```python
from build123d import *

# Parameters (mm, degrees)
F0_R     = 9
F1_DEPTH = 27.2
F2_R     = 5.5
F3_DEPTH = 23.7
F4_SIZE  = 1.5


with BuildPart() as f1:
    # F0 (on Top) → F1 (new body)
    with BuildSketch(Plane.XY):
        Circle(F0_R)
    extrude(amount=-F1_DEPTH)

    # F2 (on face) → F3 (cut)
    with BuildSketch(Plane.XY):
        Circle(F2_R)
    extrude(amount=-F3_DEPTH, mode=Mode.SUBTRACT)

    # F4
    f4_edges = [f1.edges().sort_by_distance(p)[0] for p in [
        (-9, 0, 0),
    ]]
    chamfer(f4_edges, length=F4_SIZE)


solid = f1.part
```
The listing builds one solid part. Answer for the finished solid, in the listing's coordinates (mm). A direction names the side the tool comes from. Give positions to 0.01 mm unless a question says otherwise; leave off trailing zeros. Write each loop counter-clockwise with the first axis right and the second up, starting at its lowest first coordinate (ties: lowest second). Pieces come first, ordered by that corner, then holes. Notation, with made-up numbers: (3, 39.5) - (36, 39.5) arc R24 cw to (36, 51.5) - close; hole circle Ø9 at (33, 32.5). An arc over 180 degrees is marked (long way). Use one line per item in the form item = value. Start each with the question number.
1) Find section B-B on x = 0. Determine the outline of the cut face in (y, z).
2) A tool of negligible diameter and unlimited length cuts with its end or side. For faces 1 (the face through (-1.19, -5.37, -11.68)), 2 (the face through (-4, 4, 0)), from which of +Z, -Z, +X, -X, +Y, -Y can it reach the whole face along a straight path? Write none if from no direction.
3) The mould has two halves that part along Y. Classify faces 3 (the face through (-1.172, 8.923, -14.17)), 4 (the face through (0, 0, -23.7)), 5 (the face through (0, 0, -27.2)): pulls with the +Y half, pulls with the -Y half, needs draft (parallel to the pull), parting line crosses it, or undercut.
4) Consider line 1 along Y through (x, z) = (0, -13.5); line 2 along X through (y, z) = (4.5, -7.75); line 3 along Z through (x, y) = (5, -0.25). Determine where each line is inside the solid, lowest interval first. Write a range as from..to.
5) Find section A-A on z = -3. Determine the outline of the cut face in (x, y).
6) Flat-ended cylindrical pins translate along their axes: pin 1 Ø1.5 at (x, z) = (-3.5, -7) entering from -Y; pin 2 Ø6 at (y, z) = (7, -14) entering from +X; pin 3 Ø3 at (y, z) = (7, -22) entering from +X. Find the tip coordinate at first contact, or state that the pin passes through.
Geometry results:
q1.outline = (-9, -27.2) - (9, -27.2) - (9, -1.5) - (7.5, 0) - (5.5, 0) - (5.5, -23.7) - (-5.5, -23.7) - (-5.5, 0) - (-7.5, 0) - (-9, -1.5) - close
q2.face_1 = +Z
q2.face_2 = +Z, +X, -X, +Y, -Y
q3.face_3 = parting line crosses it
q3.face_4 = undercut
q3.face_5 = needs draft
q4.line_1 = -9..-5.5, 5.5..9
q4.line_2 = -7.79..-3.16, 3.16..7.79
q4.line_3 = -27.2..-23.7
q5.outline = circle Ø18 at (0, 0); hole circle Ø11 at (0, 0)
q6.pin_1 = -8.57
q6.pin_2 = 8.06
q6.pin_3 = 7.12
